The figure shows three views and two pictorial views of one solid part (mm, origin at its lowest corner). Answer the questions. Coordinates: 2 decimals unless noted, no trailing zeros. Write each loop counter-clockwise with the first axis right and the second up, starting at its lowest first coordinate (ties: lowest second). Pieces come first, ordered by that corner, then holes. Notation, with made-up numbers: (57.5, 34) - (82.5, 34) arc R21 cw to (82.5, 52) - close; hole circle Ø4 at (-8, -25.5). An arc over 180 degrees is marked (long way). Use a Markdown table: item, result. Add a question column.
(1) Given pin 1 Ø4 at (x, y) = (9.5, 3.5) entering from -Z; pin 2 Ø9 at (y, z) = (15, 10) entering from +X, each flat-ended and moving along its own axis, determine where each tip first touches the part or whether it passes through.
(2) The part is cut by section A-A, the plane z = 25. Give the vertices of the cut face in (x, y), then the cut area to 3 significant figures.
(3) The part is cut by section C-C, the plane y = 25. Give the vertices of the cut face in (x, z).
(4) Find the intervals of material crossed by line 1 (X direction, y = 5.5, z = 109); line 2 (Y direction, x = 5.75, z = 36.5); line 3 (Y direction, x = 16.3, z = 25), in increasing order. Write a range as from..to.
(5) The part is cut by section B-B, the plane x = 8. Give the vertices of the cut face in (y, z), then the cut area to 3 significant figures.
(6) The part is cut by section D-D, the plane z = 112. Give the vertices of the cut face in (x, y), then the cut area to 3 significant figures.
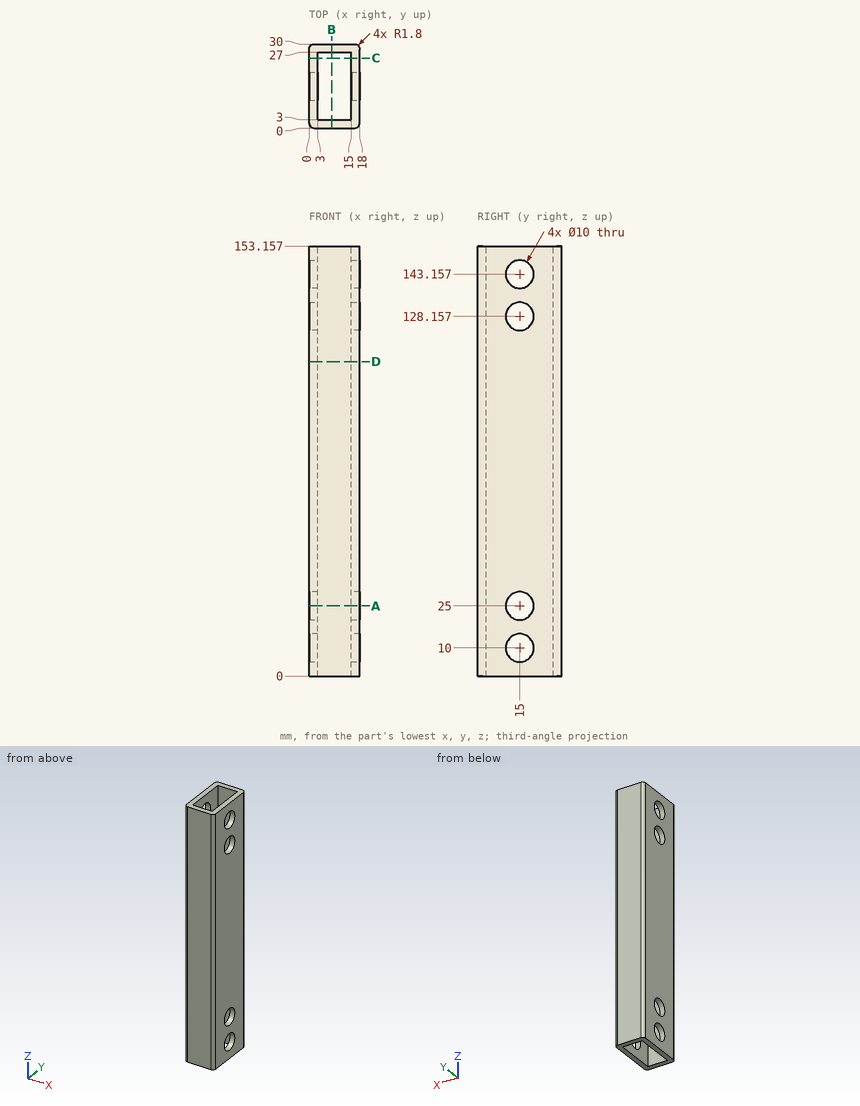
Model answer:
| question | item | result |
|---|---|---|
| 1 | pin 1 | z = 0 |
| 1 | pin 2 | through |
| 2 | outline | (0, 1.8) arc R1.8 ccw to (1.8, 0) - (16.2, 0) arc R1.8 ccw to (18, 1.8) - (18, 10) - (15, 10) - (15, 3) - (3, 3) - (3, 10) - (0, 10) - close; (0, 20) - (3, 20) - (3, 27) - (15, 27) - (15, 20) - (18, 20) - (18, 28.2) arc R1.8 ccw to (16.2, 30) - (1.8, 30) arc R1.8 ccw to (0, 28.2) - close |
| 2 | area | 189 mm^2 |
| 3 | outline | (0, 0) - (3, 0) - (3, 153.16) - (0, 153.16) - close; (15, 0) - (18, 0) - (18, 153.16) - (15, 153.16) - close |
| 4 | line 1 | 0..3, 15..18 |
| 4 | line 2 | 0..3, 27..30 |
| 4 | line 3 | 0..10, 20..30 |
| 5 | outline | (0, 0) - (3, 0) - (3, 153.16) - (0, 153.16) - close; (27, 0) - (30, 0) - (30, 153.16) - (27, 153.16) - close |
| 5 | area | 919 mm^2 |
| 6 | outline | (0, 1.8) arc R1.8 ccw to (1.8, 0) - (16.2, 0) arc R1.8 ccw to (18, 1.8) - (18, 28.2) arc R1.8 ccw to (16.2, 30) - (1.8, 30) arc R1.8 ccw to (0, 28.2) - close; hole (3, 3) - (15, 3) - (15, 27) - (3, 27) - close |
| 6 | area | 249 mm^2 |
